Source: CAD feature listing. Evaluate the final solid. Frame: model axes, mm. Face numbers are marked on the shaded views. Give positions to 0.01 mm unless a question says otherwise; leave off trailing zeros. Write each loop counter-clockwise with the first axis right and the second up, starting at its lowest first coordinate (ties: lowest second). Pieces come first, ordered by that corner, then holes. Notation, with made-up numbers: (14.5, 45) -> (20.5, 45) arc R12 cw to (20.5, 49) -> close; hole circle Ø10 at (67.25, -26.75). An arc over 180 degrees is marked (long way). Write item = value, one per line.
from build123d import *

# Parameters (mm, degrees)
F0_R     = 50
F0_R_2   = 47.5
F1_DEPTH = 101.6
F4_DEPTH = 5
F6_DEPTH = 5
F7_F1_R  = 1
F7_F2_R  = 1
F7_F3_R  = 1
F7_F4_R  = 1


# Not quite as in the source:
# - a fillet or chamfer that OpenCascade refuses, or shapes differently, is made with other operations: its cross-section is extruded or revolved along the edge and cut away or added


with BuildPart() as f1:
    # F0 (on Top) → F1 (new body)
    with BuildSketch(Plane.XY):
        Circle(F0_R)
        Circle(F0_R_2, mode=Mode.SUBTRACT)
    extrude(amount=F1_DEPTH)

    # F2: fillet of radius 5.08 on 1 edges, made by hand

    # F2_s1 → F2_t2 (revolve, cut)
    with BuildSketch(Plane.XZ):
        with BuildLine():
            ThreePointArc((50, 97.2239287026), (49.3309409427, 99.7438493363), (47.5, 101.6))
            Line((47.5, 101.6), (50, 101.6))
            Line((50, 101.6), (50, 97.2239287026))
        make_face()
    revolve(axis=Axis((0, 0, 101.6), (0, 0, 1)), mode=Mode.SUBTRACT)

    # F3: fillet of radius 5.08 on 1 edges, made by hand

    # F3_s1 → F3_t2 (revolve, cut)
    with BuildSketch(Plane.XZ):
        with BuildLine():
            ThreePointArc((50, 4.3760712974), (49.3309409427, 1.8561506637), (47.5, 0))
            Line((47.5, 0), (50, 0))
            Line((50, 0), (50, 4.3760712974))
        make_face()
    revolve(axis=Axis((0, 0, 0), (0, 0, 1)), mode=Mode.SUBTRACT)

    # F0 (on Top) → F4 (join)
    with BuildSketch(Plane.XY):
        Circle(F0_R_2)
    extrude(amount=F4_DEPTH)

    # F5 (on Front) → F6 (join, symmetric)
    with BuildSketch(Plane.XZ):
        with BuildLine():
            Line((49.9294716591, 19.3719161714), (50.0663593411, 14.3504645675))
            ThreePointArc((50.0663593411, 14.3504645675), (92.5802970628, 54.2713878676), (50.0663593411, 94.1923111677))
            Line((50.0663593411, 94.1923111677), (49.7880062733, 89.1598259546))
            ThreePointArc((49.7880062733, 89.1598259546), (87.5802251549, 54.3423353762), (49.9294716591, 19.3719161714))
        make_face()
    extrude(amount=F6_DEPTH, both=True)

    # F7: fillet of radius 1 on 4 edges, made by hand

    # F7_f1
    f7_f1_edges = [f1.edges().sort_by_distance(p)[0] for p in [
        (87.5802251549, -5, 54.3423353762),
    ]]
    fillet(f7_f1_edges, radius=F7_F1_R)

    # F7_f2
    f7_f2_edges = [f1.edges().sort_by_distance(p)[0] for p in [
        (92.5802970628, -5, 54.2713878676),
    ]]
    fillet(f7_f2_edges, radius=F7_F2_R)

    # F7_f3
    f7_f3_edges = [f1.edges().sort_by_distance(p)[0] for p in [
        (92.5802970628, 5, 54.2713878676),
    ]]
    fillet(f7_f3_edges, radius=F7_F3_R)

    # F7_f4
    f7_f4_edges = [f1.edges().sort_by_distance(p)[0] for p in [
        (87.5802251549, 5, 54.3423353762),
    ]]
    fillet(f7_f4_edges, radius=F7_F4_R)


solid = f1.part
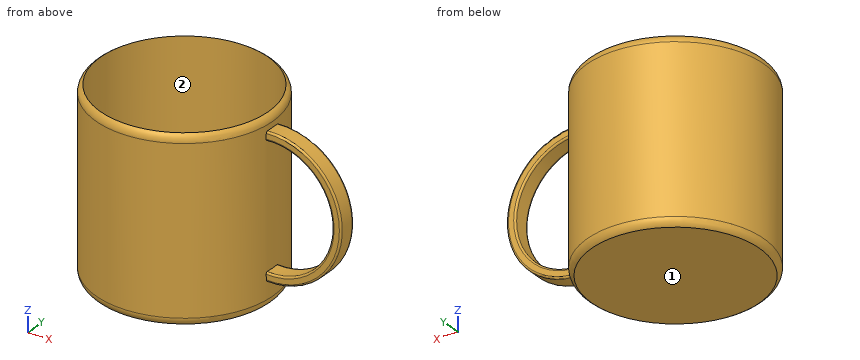
(1) Pull-direction query (X, two-part tool) for the marked faces 1 and 2; classes: pulls with the +X half, pulls with the -X half, needs draft (parallel to the pull), parting line crosses it, or undercut.
Values follow:
face_1 = needs draft
face_2 = undercut
(2) Section query A-A (x = 0). Return loops of the section in (y, z).
Values follow:
outline = (-50, 4.38) arc R5.08 ccw to (-47.5, 0) -> (47.5, 0) arc R5.08 ccw to (50, 4.38) -> (50, 97.22) arc R5.08 ccw to (47.5, 101.6) -> (47.5, 5) -> (-47.5, 5) -> (-47.5, 101.6) arc R5.08 ccw to (-50, 97.22) -> close
(3) Section query B-B (y = 0). Return loops of the section in (x, z), plus the area to 3 significant figures.
Values follow:
outline = (-50, 4.38) arc R5.08 ccw to (-47.5, 0) -> (47.5, 0) arc R5.08 ccw to (50, 4.38) -> (50, 16.78) -> (50.07, 14.35) arc R40 ccw (long way) to (50.07, 94.19) -> (50, 92.99) -> (50, 97.22) arc R5.08 ccw to (47.5, 101.6) -> (47.5, 5) -> (-47.5, 5) -> (-47.5, 101.6) arc R5.08 ccw to (-50, 97.22) -> close; hole (50, 19.37) arc R35 ccw (long way) to (50, 89.18) -> close
area = 1,580 mm2
(4) First-contact query: pin 1 (3 mm diameter, centred on y = -10.5, z = 14, fed in from +X); pin 2 (10 mm diameter, centred on x = -17, y = -18.5, fed in from -Z); pin 3 (21 mm diameter, centred on x = 79, z = 44, fed in from +Y); pin 4 (8 mm diameter, centred on y = -38, z = 47, fed in from +X). Flat tips, straight axial feed; report the tip coordinate or a pass-through.
Values follow:
pin_1 = 49.18
pin_2 = 0
pin_3 = 5
pin_4 = 36.66
(5) Section query C-C (z = 67). Give the number of separate pieces and of enclosed holes in the cut face, plus the area to 3 significant figures.
Values follow:
separate_pieces = 2
enclosed_holes = 1
area = 818 mm2
(6) Material intervals for line 1 (Y direction, x = 0, z = 44); line 2 (X direction, y = -14.5, z = 74.5); line 3 (X direction, y = -27.5, z = 63), sorted ascending.
Values follow:
line_1 = -50 to -47.5, 47.5 to 50
line_2 = -47.85 to -45.23, 45.23 to 47.85
line_3 = -41.76 to -38.73, 38.73 to 41.76
